Check sheet for the modelled part. Datum: model origin and axes. Units: mm. Face numbers are marked on the shaded views. A direction names the side the tool comes from. Coordinates: 2 decimals unless noted, no trailing zeros. Loops run counter-clockwise (first coordinate to the right, second up) from the corner with the lowest first, then second, coordinate; pieces in that order, holes last. Notation, with made-up numbers: M -32,1 L 0,1 A16 ccw 0,5 Z; hole C 14.25,-31 d4. An arc over 180 degrees is marked long. Write each question's results on one line, items separated by ' | '. Start each with the question number.
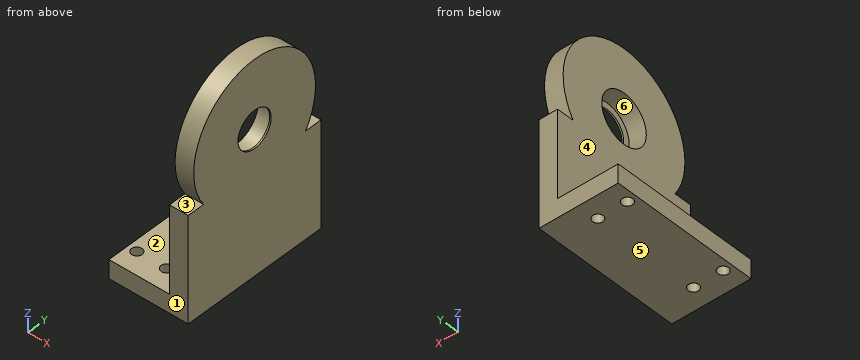
from build123d import *

# Parameters (mm, degrees)
SKETCH1_R           = 22
BOSS_EXTRUDE1_DEPTH = 6
SKETCH2_W           = 34
SKETCH2_H           = 48
BOSS_EXTRUDE2_DEPTH = 6
SKETCH3_R           = 6
CUT_EXTRUDE1_DEPTH  = 6
SKETCH4_R           = 8.05
CUT_EXTRUDE2_DEPTH  = 5.5
SKETCH5_W           = 19.51
SKETCH5_H           = 48
SKETCH5_R           = 1.7
BOSS_EXTRUDE3_DEPTH = 6


with BuildPart() as part:
    # Sketch1 → Boss-Extrude1 (new body)
    with BuildSketch(Plane(origin=(336.5, 0, 0), x_dir=(0, 0, -1), z_dir=(1, 0, 0))):
        with Locations((-300, 300)):
            Circle(SKETCH1_R)
    extrude(amount=BOSS_EXTRUDE1_DEPTH)

    # Sketch2 → Boss-Extrude2 (add)
    with BuildSketch(Plane(origin=(336.5, 0, 0), x_dir=(0, 0, -1), z_dir=(1, 0, 0))):
        with Locations((-271, 300)):
            Rectangle(SKETCH2_W, SKETCH2_H)
    extrude(amount=BOSS_EXTRUDE2_DEPTH)

    # Sketch3 → Cut-Extrude1 (cut)
    with BuildSketch(Plane(origin=(336.5, 0, 0), x_dir=(0, 0, -1), z_dir=(1, 0, 0))):
        with Locations((-300, 300)):
            Circle(SKETCH3_R)
    extrude(amount=CUT_EXTRUDE1_DEPTH, mode=Mode.SUBTRACT)

    # Sketch4 → Cut-Extrude2 (cut)
    with BuildSketch(Plane(origin=(336.5, 0, 0), x_dir=(0, 0, -1), z_dir=(1, 0, 0))):
        with Locations((-300, 300)):
            Circle(SKETCH4_R)
    extrude(amount=CUT_EXTRUDE2_DEPTH, mode=Mode.SUBTRACT)

    # Sketch5 → Boss-Extrude3 (add)
    with BuildSketch(Plane.XY.offset(254)):
        with Locations((326.755, 300)):
            Rectangle(SKETCH5_W, SKETCH5_H)
        with Locations((320, 282.7)):
            Circle(SKETCH5_R, mode=Mode.SUBTRACT)
        with Locations((320, 317.3)):
            Circle(SKETCH5_R, mode=Mode.SUBTRACT)
        with Locations((329.5, 282.7)):
            Circle(SKETCH5_R, mode=Mode.SUBTRACT)
        with Locations((329.5, 317.3)):
            Circle(SKETCH5_R, mode=Mode.SUBTRACT)
    extrude(amount=BOSS_EXTRUDE3_DEPTH)


solid = part.part
Item 1: Release check for a two-part mould opening along Z. For the marked faces 1, 2 and 3 record: +Z half, -Z half, draft (parallel to the pull), parting line (faces both ways), or undercut.
Item 2: Thickness scan on line 1 (X direction, y = 317.3, z = 257.7); line 2 (Y direction, x = 320, z = 258.45); line 3 (Z direction, x = 326, y = 298.5). Record the ranges inside material, lowest first.
Item 3: Section check D-D (z = 281). Record the cut outline in (x, y), plus the area to 3 significant figures.
Item 4: Tool access check on the marked faces 4, 5 and 6. Record the directions out of +Z, -Z, +X, -X, +Y, -Y that give a thin tool (end or side, any length) a straight path to the whole face; none if there is none.
Item 5: Depth check by flat-ended pin: P1, Ø14, axis at y = 300, z = 300, coming from the -X side; P2, Ø1.5, axis at x = 323, y = 302.5, coming from the +Z side; P3, Ø1, axis at y = 286.5, z = 289.5, coming from the -X side; P4, Ø10, axis at x = 332.5, z = 281.5, coming from the +Y side. Enter the tip coordinate at first touch or a pass-through.
Item 6: Section check C-C (y = 282.7). Record the cut outline in (x, z), plus the area to 3 significant figures.
Item 7: Section check A-A (y = 300). Record the cut outline in (x, z).
Item 8: Section check B-B (z = 300). Record the cut outline in (x, y), plus the area to 3 significant figures.
Computed values:
1) face 1: draft | face 2: +Z half | face 3: undercut
2) line 1: x = 317 to 318.3, 321.7 to 327.8, 331.2 to 342.5 | line 2: y = 276 to 281, 284.4 to 315.6, 319 to 324 | line 3: z = 254 to 260
3) outline: M 336.5,276 L 342.5,276 L 342.5,324 L 336.5,324 Z | area: 288 mm²
4) face 4: +Z, -X, +Y, -Y | face 5: -Z, +X, -X, +Y, -Y | face 6: -X
5) P1: stops at x = 342 | P2: stops at z = 260 | P3: stops at x = 336.5 | P4: stops at y = 324
6) outline: M 317,254 L 318.3,254 L 318.3,260 L 317,260 Z; M 321.7,254 L 327.8,254 L 327.8,260 L 321.7,260 Z; M 331.2,254 L 342.5,254 L 342.5,313.59 L 336.5,313.59 L 336.5,260 L 331.2,260 Z | area: 434 mm²
7) outline: M 317,254 L 342.5,254 L 342.5,294 L 342,294 L 342,291.95 L 336.5,291.95 L 336.5,260 L 317,260 Z; M 336.5,308.05 L 342,308.05 L 342,306 L 342.5,306 L 342.5,322 L 336.5,322 Z
8) outline: M 336.5,278 L 342.5,278 L 342.5,294 L 342,294 L 342,291.95 L 336.5,291.95 Z; M 336.5,308.05 L 342,308.05 L 342,306 L 342.5,306 L 342.5,322 L 336.5,322 Z | area: 169 mm²
